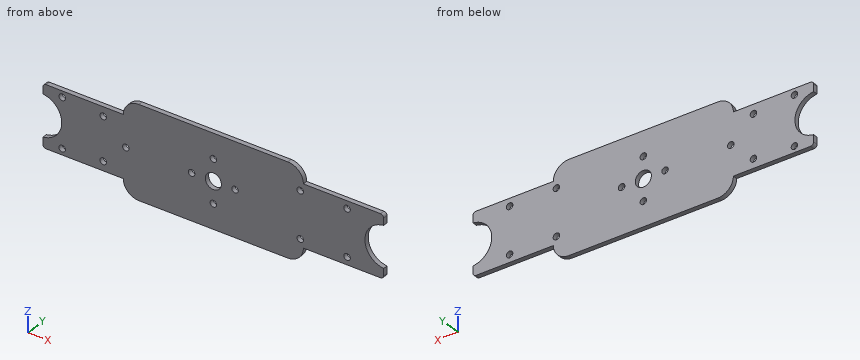
Autodesk Inventor part; units mm, degrees
ref_plane "YZ Plane" through (0, 0, 0) normal (1, 0, 0) x (0, 1, 0)
ref_plane "XZ Plane" through (0, 0, 0) normal (0, 1, 0) x (-1, 0, 0)
ref_plane "XY Plane" through (0, 0, 0) normal (0, 0, 1) x (1, 0, 0)
sketch "Sketch1" plane through (0, 0, 0) normal (0, 1, 0) x (-1, 0, 0)
  line L0 (-0.4496, -30) -> (-0.4496, 0)
  line L1 (-41.2289, 0) -> (-41.2289, -30)
  circle A0 centre (-48.8686, -22.525) radius 1.05
  circle A1 centre (-48.8686, -7.475) radius 1.05
  circle A2 centre (-63.9686, -22.525) radius 1.05
  circle A3 centre (-63.9686, -7.475) radius 1.05
  circle A4 centre (27.89, -23) radius 1.05
  circle A5 centre (27.89, -7) radius 1.05
  circle A6 centre (14.67, -22) radius 1.05
  circle A7 centre (14.67, -8) radius 1.05
  circle A8 centre (7.37, -15) radius 1.05
  circle A9 centre (-20.8393, -15) radius 2.6
  circle A10 centre (-27.8393, -15) radius 1.05
  circle A11 centre (-20.8393, -8) radius 1.05
  circle A12 centre (-20.8393, -22) radius 1.05
  circle A13 centre (-13.8393, -15) radius 1.05
  arc A14 (-75.7686, -21.7136) -> (-75.7686, -8.2864) centre (-76.4686, -15) ccw
  line L2 (-75.7686, -24) -> (-75.7686, -21.7136)
  arc A15 (-75.7686, -24) -> (-74.7686, -25) centre (-74.7686, -24) ccw
  line L3 (-74.7686, -25) -> (-49.8686, -25)
  arc A16 (-49.8686, -25) -> (-44.8686, -30) centre (-44.8686, -25) ccw
  line L4 (3.19, -30) -> (-44.8686, -30)
  arc A17 (3.19, -30) -> (8.19, -25) centre (3.19, -25) ccw
  line L5 (8.19, -25) -> (33.09, -25)
  arc A18 (33.09, -25) -> (34.09, -24) centre (33.09, -24) ccw
  line L6 (34.09, -21.7136) -> (34.09, -24)
  arc A19 (34.09, -8.2864) -> (34.09, -21.7136) centre (34.79, -15) ccw
  line L7 (34.09, -6) -> (34.09, -8.2864)
  arc A20 (34.09, -6) -> (33.09, -5) centre (33.09, -6) ccw
  line L8 (33.09, -5) -> (8.19, -5)
  arc A21 (8.19, -5) -> (3.19, 0) centre (3.19, -5) ccw
  line L9 (-44.8686, 0) -> (3.19, 0)
  arc A22 (-44.8686, 0) -> (-49.8686, -5) centre (-44.8686, -5) ccw
  line L10 (-49.8686, -5) -> (-74.7686, -5)
  arc A23 (-74.7686, -5) -> (-75.7686, -6) centre (-74.7686, -6) ccw
  line L11 (-75.7686, -8.2864) -> (-75.7686, -6)
  line L12 (-41.6786, -30) -> (-41.6786, 0)
  line L13 (-40.7793, 0) -> (-40.7793, -30)
  line L14 (-0.8993, -30) -> (-0.8993, 0)
  line L15 (0, 0) -> (0, -30)
extrude "Extrusion1" add sketch "Sketch1" against normal blind 1.5
properties part number "axis_13_top_frame"
Geometry check sheet. Reference: the model listing, model coordinates, mm. Give positions to 0.01 mm unless a question says otherwise; leave off trailing zeros. Loops run counter-clockwise (first coordinate to the right, second up) from the corner with the lowest first, then second, coordinate; pieces in that order, holes last. Notation, with made-up numbers: M -13.75,88.25 L 22.25,88.25 A16 cw 22.25,109.25 Z; hole C 60,14.5 d9. An arc over 180 degrees is marked long. Answer as a JSON object with one key per item and string values. Group by question number.
Item 1: Gauge pin test, flat ends, axial feed: pin 1 (0.8 mm diameter, centred on x = 68.5, y = -0.5, fed in from +Z); pin 2 (0.8 mm diameter, centred on x = 57, y = -0.5, fed in from -Z); pin 3 (1.3 mm diameter, centred on x = -7.37, z = -15, fed in from -Y). Record the tip position at first contact, or that the pin passes through.
Item 2: Material ranges on L1, parallel to Z at x = 69.5, y = -0.3; L2, parallel to X at y = -0.5, z = -17; L3, parallel to X at y = -1.35, z = -28.5, recorded low to high.
Item 3: Sectioned sample at C-C on z = -27. Record the boundary of the cut face in (x, y).
Item 4: Sectioned sample at A-A on y = -0.5. Give the number of separate pieces and of enclosed holes in the cut face, plus the area to 3 significant figures.
Item 5: Sectioned sample at B-B on x = 52.5. Record the boundary of the cut face in (y, z).
Findings below:
{
 "1": {"pin 1": "z = -5", "pin 2": "z = -25", "pin 3": "through"},
 "2": {"L1": "-25 to -5", "L2": "-28.34 to 19.18, 22.5 to 70.02", "L3": "-6.76 to 48.44"},
 "3": {"outline": "M -7.77,-1.5 L 49.45,-1.5 L 49.45,0 L -7.77,0 Z"},
 "4": {"separate pieces": "1", "enclosed holes": "14", "area": "2,560 mm2"},
 "5": {"outline": "M -1.5,-25 L 0,-25 L 0,-5 L -1.5,-5 Z"}
}
